Work out the finished part from the listing and answer in its coordinate system (mm). A direction names the side the tool comes from. Round coordinates to 2 decimals unless told otherwise and drop trailing zeros. Loops run counter-clockwise (first coordinate to the right, second up) from the corner with the lowest first, then second, coordinate; pieces in that order, holes last.
```python
from build123d import *

# Parameters (mm, degrees)
SKETCH_1_R          = 8
EXTRUDE_1_DEPTH     = 0.65
EXTRUDE_START       = 0.65
SKETCH_2_R          = 6.07
SKETCH_2_R_2        = 5.1
EXTRUDE_2_DEPTH     = 0.85
CUT_EXTRUDE_START   = 0.65
SKETCH_3_R          = 5.1
CUT_EXTRUDE_1_DEPTH = 0.01
SKETCH_4_W          = 6.9
SKETCH_4_H          = 6.9
CUT_EXTRUDE_2_DEPTH = 0.64
CHAMFER_1_SIZE      = 0.3
SKETCH_6_R          = 0.207363545
CUT_EXTRUDE_3_DEPTH = 0.64


with BuildPart() as part:
    # 草图1 → 凸台-拉伸1 (new body)
    with BuildSketch(Plane.XY):
        Circle(SKETCH_1_R)
    extrude(amount=EXTRUDE_1_DEPTH)

    # 草图2 → 凸台-拉伸2 (add)
    with BuildSketch(Plane.XY.offset(EXTRUDE_START)):
        Circle(SKETCH_2_R)
        Circle(SKETCH_2_R_2, mode=Mode.SUBTRACT)
    extrude(amount=EXTRUDE_2_DEPTH)

    # 草图3 → 切除-拉伸1 (cut)
    with BuildSketch(Plane.XY.offset(CUT_EXTRUDE_START)):
        Circle(SKETCH_3_R)
    extrude(amount=-CUT_EXTRUDE_1_DEPTH, mode=Mode.SUBTRACT)

    # 草图4 → 切除-拉伸2 (cut)
    with BuildSketch(Plane.XY):
        Rectangle(SKETCH_4_W, SKETCH_4_H)
    extrude(amount=CUT_EXTRUDE_2_DEPTH, mode=Mode.SUBTRACT)

    # 倒角1
    chamfer_1_edges = [part.edges().sort_by_distance(p)[0] for p in [
        (-5.1, 0, 1.5),
    ]]
    chamfer(chamfer_1_edges, length=CHAMFER_1_SIZE)

    # 草图6 → 切除-拉伸3 (cut)
    with BuildSketch(Plane.XY):
        with Locations((-3.45, 3.45)):
            Circle(SKETCH_6_R)
        with Locations((3.45, 3.45)):
            Circle(SKETCH_6_R)
        with Locations((3.45, -3.45)):
            Circle(SKETCH_6_R)
        with Locations((-3.45, -3.45)):
            Circle(SKETCH_6_R)
    extrude(amount=CUT_EXTRUDE_3_DEPTH, mode=Mode.SUBTRACT)


solid = part.part
```
1. Which of the six approach directions +Z, -Z, +X, -X, +Y, -Y give full straight-line access (tool end or side, diameter ignored) to faces 1 (the face through (-6, 2, 0.65)), 2 (the face through (0, 4, 0))?
Answer key:
face 1: +Z
face 2: -Z, +X, -X, +Y, -Y
2. Determine the mould class of faces 3 (the face through (0, -4, 0.64)), 4 (the face through (-1.73, -7.81, 0.32)), 5 (the face through (-4, -4, 1.5)) for opening direction Y: +Y half, -Y half, draft (parallel to the pull), parting line (faces both ways), or undercut.
Answer key:
face 3: undercut
face 4: parting line
face 5: draft
3. Find section C-C (z = 0.9). Write down the section's boundary in (x, y), then the cut area to 3 significant figures.
Answer key:
outline: circle Ø12.14 at (0, 0); hole circle Ø10.2 at (0, 0)
area: 34.0 mm2
4. Consider probe 1 along Y at (x, z) = (0, 0.85); probe 2 along Y at (x, z) = (-3.5, 0.3); probe 3 along Z at (x, y) = (4.25, -4.5). Determine where each line is inside the solid, lowest interval first.
Answer key:
probe 1: y = -6.07 to -5.1, 5.1 to 6.07
probe 2: y = -7.19 to -3.65, -3.25 to 3.25, 3.65 to 7.19
probe 3: z = 0 to 0.65
5. Find section D-D (x = 7.25). Write down the section's boundary in (y, z), then the cut area to 3 significant figures.
Answer key:
outline: (-3.38, 0) - (3.38, 0) - (3.38, 0.65) - (-3.38, 0.65) - close
area: 4.40 mm2
6. Find section A-A (x = 0). Write down the section's boundary in (y, z).
Answer key:
outline: (-8, 0) - (-3.45, 0) - (-3.45, 0.64) - (-5.1, 0.64) - (-5.1, 1.2) - (-5.4, 1.5) - (-6.07, 1.5) - (-6.07, 0.65) - (-8, 0.65) - close; (3.45, 0) - (8, 0) - (8, 0.65) - (6.07, 0.65) - (6.07, 1.5) - (5.4, 1.5) - (5.1, 1.2) - (5.1, 0.64) - (3.45, 0.64) - close
7. Given pin 1 (8 mm diameter, centred on x = -0.5, y = 0.5, fed in from +Z); pin 2 (0.7 mm diameter, centred on y = 1, z = 0.5, fed in from +X); pin 3 (0.7 mm diameter, centred on x = 1.5, z = 0.5, fed in from -Y), each flat-ended and moving along its own axis, determine where each tip first touches the part or whether it passes through.
Answer key:
pin 1: stops at z = 0.64
pin 2: stops at x = 7.97
pin 3: stops at y = -7.92
